Input: part model. Units: mm. Frame: model coordinates. A direction names the side the tool comes from. Coordinates: 2 decimals unless noted, no trailing zeros. Order: outer loops, then holes, each group sorted by start corner. A loop starts at its lowest first (then second) coordinate and runs counter-clockwise, first axis right, second up. Notation, with made-up numbers: (-1, 17) -> (9, 17) arc R23 cw to (9, 32) -> close; hole circle Ø6 at (5, 69). An arc over 180 degrees is marked (long way). Write each question's results on one line, items separated by ' | '.
```python
from build123d import *

# Parameters (mm, degrees)
SKETCH2_R           = 2.4
BOSS_EXTRUDE1_DEPTH = 6
SKETCH3_R           = 15
BOSS_EXTRUDE2_DEPTH = 2.5
FILLET1_R           = 2
CUT_EXTRUDE1_DEPTH  = 1.5
SKETCH5_R           = 2.5
CUT_EXTRUDE2_DEPTH  = 23.338307904
CHAMFER1_SIZE       = 0.5
CHAMFER1_SIZE2      = 0.595876796


with BuildPart() as part:
    # Sketch2 → Boss-Extrude1 (new body)
    with BuildSketch(Plane.XY):
        Circle(SKETCH2_R)
    extrude(amount=BOSS_EXTRUDE1_DEPTH)

    # Sketch3 → Boss-Extrude2 (add)
    with BuildSketch(Plane.XY.offset(6)):
        Circle(SKETCH3_R)
    extrude(amount=BOSS_EXTRUDE2_DEPTH)

    # Fillet1
    fillet1_edges = [part.edges().sort_by_distance(p)[0] for p in [
        (-2.4, 0, 6),
    ]]
    fillet(fillet1_edges, radius=FILLET1_R)

    # Sketch4 → Cut-Extrude1 (cut)
    with BuildSketch(Plane.XY.offset(8.5)):
        with BuildLine():
            ThreePointArc((0, 14.1), (-5.1, 9), (0, 3.9))
            Line((0, 3.9), (0, 14.1))
        make_face()
        with BuildLine():
            Line((0, 14.1), (0, 3.9))
            ThreePointArc((0, 3.9), (3.606244584, 5.393755416), (5.1, 9))
            ThreePointArc((5.1, 9), (3.606244584, 12.606244584), (0, 14.1))
        make_face()
        with BuildLine():
            ThreePointArc((0, -3.9), (-5.1, -9), (0, -14.1))
            Line((0, -14.1), (0, -3.9))
        make_face()
        with BuildLine():
            Line((0, -3.9), (0, -14.1))
            ThreePointArc((0, -14.1), (3.606244584, -12.606244584), (5.1, -9))
            ThreePointArc((5.1, -9), (3.606244584, -5.393755416), (0, -3.9))
        make_face()
    extrude(amount=-CUT_EXTRUDE1_DEPTH, mode=Mode.SUBTRACT)

    # Sketch5 → Cut-Extrude2 (cut, through all)
    with BuildSketch(Plane.XY.offset(7)):
        with Locations((0, -9)):
            Circle(SKETCH5_R)
        with Locations((0, 9)):
            Circle(SKETCH5_R)
    extrude(amount=-CUT_EXTRUDE2_DEPTH, mode=Mode.SUBTRACT)

    # Chamfer1
    chamfer1_edges = [part.edges().sort_by_distance(p)[0] for p in [
        (-2.4, 0, 0),
    ]]
    chamfer1_side = [part.faces().sort_by_distance(p)[0] for p in [
        (0, 0, 0),
    ]]
    chamfer(chamfer1_edges, length=CHAMFER1_SIZE, length2=CHAMFER1_SIZE2, reference=chamfer1_side[0])


solid = part.part
```
(1) Cut plane D-D, the plane z = 2.75. Return loops of the section in (x, y), plus the area to 3 significant figures.
Return value:
outline: circle Ø4.8 at (0, 0) | area: 18.1 mm2
(2) Mould query, pull axis Y, two halves, no side actions, for faces 1 (the face through (0, 0, 8.5)), 2 (the face through (-0.54, 6.56, 6.51)), 3 (the face through (1.29, 2.024, 2.274)). Classes: +Y half, -Y half, draft (parallel to the pull), parting line (faces both ways), or undercut.
Return value:
face 1: draft | face 2: undercut | face 3: parting line
(3) Cut plane C-C, the plane x = 1.5. Count the separate pieces of the cut face and the enclosed holes in it, plus the area to 3 significant figures.
Return value:
separate pieces: 3 | enclosed holes: 0 | area: 61.5 mm2
(4) Pin query (flat end, axial travel): P1, Ø15, axis at x = 4, y = -3.5, coming from the -Z side; P2, Ø6.5, axis at x = 0, y = 9, coming from the -Z side; P3, Ø3, axis at y = -0.5, z = 3, coming from the +X side; P4, Ø6, axis at x = 1.5, y = -10, coming from the +Z side. Return the tip coordinate at first contact, or that it passes through.
Return value:
P1: z = 0 | P2: z = 6 | P3: x = 2.45 | P4: z = 7
(5) Line query: line 1 along Y through (x, z) = (0, 6.6); line 2 along Z through (x, y) = (-9.75, -0.75); line 3 along Y through (x, z) = (1.75, 6.25). Output: solid intervals per line, ascending. Write a range as from..to.
Return value:
line 1: -15..-11.5, -6.5..6.5, 11.5..15 | line 2: 6..8.5 | line 3: -14.9..-10.79, -7.21..7.21, 10.79..14.9
(6) Cut plane A-A, the plane y = 0. Return loops of the section in (x, z), plus the area to 3 significant figures.
Return value:
outline: (-15, 6) -> (-4.4, 6) arc R2 cw to (-2.4, 4) -> (-2.4, 0.6) -> (-1.9, 0) -> (1.9, 0) -> (2.4, 0.6) -> (2.4, 4) arc R2 cw to (4.4, 6) -> (15, 6) -> (15, 8.5) -> (-15, 8.5) -> close | area: 105 mm2
(7) Cut plane B-B, the plane y = 8. Return loops of the section in (x, z).
Return value:
outline: (-12.69, 6) -> (-2.29, 6) -> (-2.29, 7) -> (-5, 7) -> (-5, 8.5) -> (-12.69, 8.5) -> close; (2.29, 6) -> (12.69, 6) -> (12.69, 8.5) -> (5, 8.5) -> (5, 7) -> (2.29, 7) -> close
(8) Reachability of faces 4 (the face through (-4, -3, 6)), 5 (the face through (0, 0, 0)) from +Z, -Z, +X, -X, +Y, -Y: full face, straight path, thin tool, end or side. Return the list, or none.
Return value:
face 4: -Z | face 5: -Z, +X, -X, +Y, -Y
